from build123d import *

# Parameters (mm, degrees)
PAD002_DEPTH    = 2
PAD003_DEPTH    = 4.9
POCKET005_DEPTH = 4.1
POCKET006_DEPTH = 11
SKETCH011_W     = 10
SKETCH011_H     = 3.5
POCKET007_DEPTH = 5
PAD004_DEPTH    = 1.4
PAD006_DEPTH    = 2
SKETCH013_R     = 0.925
POCKET009_DEPTH = 5
CHAMFER_SIZE    = 0.5
CHAMFER001_SIZE = 0.5
CHAMFER006_SIZE = 0.3


with BuildPart() as part:
    # Sketch008 (on Face1 of ReferencePocket001) → Pad002 (new body)
    with BuildSketch(Plane.XY.offset(3.9)):
        with BuildLine():
            Line((0.05, 0.05), (18.15, 0.05))
            Line((18.15, 0.05), (18.15, 26.100026))
            ThreePointArc((18.15, 26.100026), (9.1, 35.150026), (0.05, 26.100026))
            Line((0.05, 0.05), (0.05, 26.100026))
        make_face()
        with BuildLine():
            Line((0.65, 0.65), (17.55, 0.65))
            Line((17.55, 0.65), (17.55, 26.100026))
            ThreePointArc((17.55, 26.100026), (9.1, 34.550026), (0.65, 26.100026))
            Line((0.65, 0.65), (0.65, 26.100026))
        make_face(mode=Mode.SUBTRACT)
    extrude(amount=-PAD002_DEPTH)

    # Sketch009 (on Face9 of Pad002) → Pad003 (join)
    with BuildSketch(Plane.XY.offset(3.9)):
        with BuildLine():
            Line((-0.86, -0.86), (19.06, -0.86))
            Line((19.06, -0.86), (19.06, 26.10003))
            ThreePointArc((19.06, 26.10003), (9.1, 36.060031), (-0.86, 26.100031))
            Line((-0.86, -0.86), (-0.86, 26.100031))
        make_face()
    extrude(amount=PAD003_DEPTH)

    # Pad003 Face16 → Pocket005 (cut)
    with BuildSketch(Plane(origin=(9.1, 16.748749, 3.9), x_dir=(0, -1, 0), z_dir=(0, 0, -1))):
        with BuildLine():
            Line((16.098749, 8.45), (-9.351278, 8.45))
            ThreePointArc((-9.351278, 8.45), (-17.801278, 0), (-9.351278, -8.45))
            Line((-9.351278, -8.45), (16.098749, -8.45))
            Line((16.098749, -8.45), (16.098749, 8.45))
        make_face()
    extrude(amount=-POCKET005_DEPTH, mode=Mode.SUBTRACT)

    # Sketch010 (on Face8 of Pocket005) → Pocket006 (cut)
    with BuildSketch(Plane.YZ.offset(18.15)):
        Polygon((0.66, 1.9), (5.05, 1.9), (20.05, 1.9), (20.05, 2.4), (5.05, 2.4), (5.05, 5.5), (0.66, 5.5), (0.66, 1.8), (0.05, 1.8), (0.05, 1.9), align=None)
    extrude(amount=-POCKET006_DEPTH, mode=Mode.SUBTRACT)

    # Sketch011 (on Face4 of Pad002) → Pocket007 (cut)
    with BuildSketch(Plane(origin=(0.05, 0, 0), x_dir=(0, -1, 0), z_dir=(-1, 0, 0))):
        with Locations((-14, 1.75)):
            Rectangle(SKETCH011_W, SKETCH011_H)
    extrude(amount=-POCKET007_DEPTH, mode=Mode.SUBTRACT)

    # Sketch012 (on Face4 of Pad002) → Pad004 (join, symmetric)
    with BuildSketch(Plane(origin=(9.05, 0, 0), x_dir=(0, -1, 0), z_dir=(-1, 0, 0))):
        Polygon((-0.05, 2.1), (0.25, 2.4), (0.25, 2.8), (-0.05, 3.1), align=None)
        Polygon((-35.450026, 2.4), (-35.450026, 2.8), (-35.150026, 3.1), (-34.650026, 3.1), (-34.650026, 2.1), (-35.150026, 2.1), align=None)
    extrude(amount=PAD004_DEPTH, both=True)

    # Sketch014 (on Face47 of Pad004) → Pad006 (join)
    with BuildSketch(Plane(origin=(0, 0, 8), x_dir=(1, 0, 0), z_dir=(0, 0, -1))):
        with BuildLine():
            Line((17.55, -26.100026), (17.55, -17.081305))
            Line((17.55, -17.081305), (16.25, -17.081305))
            Line((16.25, -17.081305), (16.25, -21.596694))
            ThreePointArc((17.55, -26.100026), (17.218497, -23.756418), (16.25, -21.596694))
        make_face()
        with BuildLine():
            Line((0.65, -26.100026), (0.65, -17.081305))
            Line((0.65, -17.081305), (1.95, -17.081305))
            Line((1.95, -17.081305), (1.95, -21.596694))
            ThreePointArc((1.95, -21.596694), (0.981503, -23.756418), (0.65, -26.100026))
        make_face()
    extrude(amount=PAD006_DEPTH)

    # Sketch013 (on Face20 of Pocket005) → Pocket009 (cut, symmetric)
    with BuildSketch(Plane(origin=(0, 0, 8), x_dir=(1, 0, 0), z_dir=(0, 0, -1))):
        with Locations((1.525, -20.081305)):
            Circle(SKETCH013_R)
        with Locations((16.675, -20.081305)):
            Circle(SKETCH013_R)
    extrude(amount=POCKET009_DEPTH, both=True, mode=Mode.SUBTRACT)

    # Chamfer
    chamfer_edges = [part.edges().sort_by_distance(p)[0] for p in [
        (9.1, -0.86, 3.9),
    ]]
    chamfer(chamfer_edges, length=CHAMFER_SIZE)

    # Chamfer001
    chamfer001_edges = [part.edges().sort_by_distance(p)[0] for p in [
        (-0.86, 12.620015, 8.8),
        (9.1, 36.060031, 8.8),
        (19.06, 12.620015, 8.8),
        (9.1, -0.86, 8.8),
    ]]
    chamfer(chamfer001_edges, length=CHAMFER001_SIZE)

    # Chamfer006
    chamfer006_edges = [part.edges().sort_by_distance(p)[0] for p in [
        (15.75, 20.081305, 8.8),
        (0.6, 20.081305, 8.8),
    ]]
    chamfer(chamfer006_edges, length=CHAMFER006_SIZE)


solid = part.part
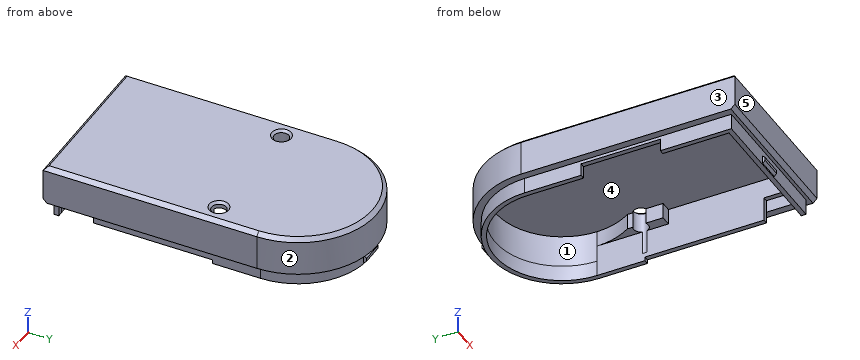
Model file for the job. Use its own axes, mm. Face numbers are marked on the shaded views. A direction names the side the tool comes from. Give positions to 0.01 mm unless a question says otherwise; leave off trailing zeros. Order: outer loops, then holes, each group sorted by start corner. A loop starts at its lowest first (then second) coordinate and runs counter-clockwise, first axis right, second up. Notation, with made-up numbers: M -11.5,3.5 L 27.5,3.5 A23 ccw 27.5,42.5 Z; hole C 67.5,-27.75 d6. An arc over 180 degrees is marked long. Put each result on its own line as item: value. Start each with the question number.
(1) Drill centre lines: L1, parallel to X at y = 25, z = 3.5; L2, parallel to X at y = 20.5, z = 5; L3, parallel to Y at x = 16.5, z = 7.75. Where is each one in solid material? Low to high. Write a range as [from, to].
(2) Band-saw the part on B-B on y = 24. Give the cut face in (x, z), then the cut area to 3 significant figures.
(3) Band-saw the part on A-A on y = 6.5. Give the cut face in (x, z), then the cut area to 3 significant figures.
(4) Tool access for the marked faces 1 and 2: list every direction of +Z, -Z, +X, -X, +Y, -Y with a clear straight run to the whole face (end or side of a thin tool).
(5) Pin check, flat tips, straight feed: pin 1 Ø1.5 at (x, z) = (5, 6.5) entering from +Y; pin 2 Ø0.5 at (x, y) = (18, 11.5) entering from -Z; pin 3 Ø1.8 at (x, z) = (12.5, 6.5) entering from +Y; pin 4 Ø2 at (y, z) = (17, 3.5) entering from -X. Stop position of each tip, or through.
(6) Pull direction Y, two halves, no side cores. Call the marked faces 3, 4 and 5: released by +Y, released by -Y, zero draft, split by the parting line, or undercut.
Results below:
1. L1: x = [0.05, 0.65], [17.55, 18.15]
1. L2: x = [-0.86, 0.65], [17.55, 19.06]
1. L3: y = [-0.86, 0.65], [17.08, 19.17], [20.99, 22.02], [30.18, 32.77]
2. outline: M -0.86,3.9 L 0.05,3.9 L 0.05,1.9 L 0.65,1.9 L 0.65,6 L 0.92,6 L 0.92,8 L 17.28,8 L 17.28,6 L 17.55,6 L 17.55,1.9 L 18.15,1.9 L 18.15,3.9 L 19.06,3.9 L 19.06,8.3 L 18.56,8.8 L -0.36,8.8 L -0.86,8.3 Z
2. area: 31.5 mm2
3. outline: M -0.86,3.9 L 0.05,3.9 L 0.05,1.9 L 0.65,1.9 L 0.65,8 L 17.55,8 L 17.55,2.4 L 18.15,2.4 L 18.15,3.9 L 19.06,3.9 L 19.06,8.3 L 18.56,8.8 L -0.36,8.8 L -0.86,8.3 Z
3. area: 30.2 mm2
4. face 1: -Z
4. face 2: +Z, -Z, +Y
5. pin 1: stops at y = 35.48
5. pin 2: stops at z = 2.4
5. pin 3: stops at y = 35.74
5. pin 4: stops at x = -0.86
6. face 3: zero draft
6. face 4: undercut
6. face 5: released by -Y
